Check sheet for the modelled part. Datum: model origin and axes. Units: mm. A direction names the side the tool comes from. Give positions to 0.01 mm unless a question says otherwise; leave off trailing zeros. Order: outer loops, then holes, each group sorted by start corner. A loop starts at its lowest first (then second) coordinate and runs counter-clockwise, first axis right, second up.
Autodesk Inventor part; units mm, degrees
ref_plane "YZ Plane" through (0, 0, 0) normal (1, 0, 0) x (0, 1, 0)
ref_plane "XZ Plane" through (0, 0, 0) normal (0, 1, 0) x (-1, 0, 0)
ref_plane "XY Plane" through (0, 0, 0) normal (0, 0, 1) x (1, 0, 0)
sketch "스케치1" plane through (0, 0, 0) normal (0, 1, 0) x (-1, 0, 0)
  line L0 (-21.65, 75) -> (21.65, 75)
  line L1 (21.65, 75) -> (21.65, -75)
  line L2 (21.65, -75) -> (-21.65, -75)
  line L3 (-21.65, -75) -> (-21.65, 75)
  line L4 (-21.65, 75) -> (21.65, -75) construction
  line L5 (21.65, 75) -> (-21.65, -75) construction
  line L6 (-21.65, 7) -> (21.65, 7)
  point P0 (0, 0)
  dimension "d0" = 43.3
  dimension "d1" = 150
  dimension "d2" = 68
extrude "돌출2" add sketch "스케치1" along normal blind 5 contours L0 L1 L6 L3
extrude "돌출3" add sketch "스케치1" along normal blind 8.5 contours L6 L1 L2 L3
sketch "스케치3" plane through (0, 8.5, 0) normal (0, 1, 0) x (1, 0, 0)
  line L0 (-21.65, -7) -> (21.65, -7)
  line L1 (21.65, 75) -> (-21.65, 75)
  line L2 (6.1, -7) -> (-6.1, -7)
  line L3 (-6.1, -7) -> (-6.1, 75)
  line L4 (-6.1, 75) -> (6.1, 75)
  line L5 (6.1, 75) -> (6.1, -7)
  line L6 (21.65, -7) -> (21.65, 75)
  line L7 (21.65, 75) -> (6.1, 75)
  line L8 (6.1, 75) -> (6.1, -7)
  line L9 (6.1, -7) -> (21.65, -7)
  line L10 (21.65, -7) -> (21.65, 75)
  line L11 (-21.65, 75) -> (-6.1, 75)
  line L12 (-6.1, 75) -> (-6.1, -7)
  line L13 (-6.1, -7) -> (-21.65, -7)
  line L14 (-21.65, -7) -> (-21.65, 75)
  point P0 (0, 0)
  point P1 (-6.1, -7)
  point P2 (6.1, 75)
  dimension "d9" = 12.2
  dimension "d11" = 6.1
extrude "돌출4" add sketch "스케치3" along normal blind 12.2 contours L14 L1 L3 L0 | L5 L1 L6 L0
sketch "스케치4" plane through (0, 5, 0) normal (0, 1, 0) x (1, 0, 0)
  line L0 (16.55, -19.1) -> (16.55, -62.7) construction
  line L1 (14.55, -21.1) -> (14.55, -60.7)
  line L2 (18.55, -60.7) -> (18.55, -21.1)
  arc A0 (18.55, -21.1) -> (14.55, -21.1) centre (16.55, -21.1) ccw
  arc A1 (14.55, -60.7) -> (18.55, -60.7) centre (16.55, -60.7) ccw
  line L3 (21.65, -75) -> (21.65, -7)
  line L4 (-21.65, -75) -> (21.65, -75)
  line L5 (21.65, -7) -> (-21.65, -7)
  line L6 (0, -7) -> (0, -75)
  line L7 (-16.55, -19.1) -> (-16.55, -62.7) construction
  line L8 (-14.55, -21.1) -> (-14.55, -60.7)
  line L9 (-18.55, -60.7) -> (-18.55, -21.1)
  arc A2 (-14.55, -21.1) -> (-18.55, -21.1) centre (-16.55, -21.1) ccw
  arc A3 (-18.55, -60.7) -> (-14.55, -60.7) centre (-16.55, -60.7) ccw
  point P0 (0, 0)
  point P1 (16.55, -40.9)
  point P2 (-16.55, -40.9)
  dimension "d14" = 43.6
  dimension "d15" = 3.1
  dimension "d16" = 4
  dimension "d17" = 12.3
extrude "돌출5" cut sketch "스케치4" against normal through all contours A0 L2 A1 L1 | L8 A3 L9 A2
fillet "모깎기1" radius 4.5 2 edges at (21.65, 2.5, 75) (-21.65, 2.5, 75)
sketch "스케치5" plane through (-21.65, 5, 7) normal (0, 0, 1) x (1, 0, 0)
  line L0 (27.75, 3.5) -> (15.55, 3.5)
  line L1 (21.65, 3.5) -> (21.65, 29.9168)
  line L2 (43.3, 0) -> (43.3, 15.7)
  line L3 (4.5, 0) -> (38.8, 0)
  line L4 (43.3, 15.7) -> (27.75, 15.7)
  line L5 (27.75, 15.7) -> (27.75, 0)
  line L6 (27.75, 0) -> (43.3, 0)
  line L7 (43.3, 0) -> (43.3, 15.7)
  line L8 (43.3, 0) -> (29.75, 15.7)
  line L9 (43.3, 15.7) -> (27.75, 15.7)
  line L10 (43.3, -5) -> (38.8, -5)
  line L11 (0, 0) -> (0, 15.7)
  line L12 (0, 15.7) -> (15.55, 15.7)
  line L13 (0, 0) -> (0, 15.7)
  line L14 (0, 0) -> (13.55, 15.7)
  point P0 (21.65, -5)
  dimension "d21" = 2
  dimension "d22" = 5
extrude "돌출6" cut sketch "스케치5" against normal through all contours L8 L4 L2 | L11 L12 L14
sketch "스케치7" plane through (-21.65, 5, -75) normal (-0.757, 0.6534, 0) x (0, 0, 1)
  line L0 (0, 20.7387) -> (82, 20.7387)
  line L1 (82, 0) -> (0, 0)
  line L2 (82, 20.7387) -> (82, 0)
  circle A0 centre (10, 9.7387) radius 1.75
  line L3 (82, 28.2909) -> (82, 0)
  line L4 (82, 9.7387) -> (0, 9.7387)
  line L5 (0, 24.5057) -> (0, -3.7852)
  line L6 (82, 20.7806) -> (0, 20.7806)
  line L7 (41, 20.7806) -> (41, 0)
  circle A1 centre (72, 9.7387) radius 1.75
  dimension "d26" = 3.5
  dimension "d28" = 10
  dimension "d39" = 11
extrude "돌출7" cut sketch "스케치7" against normal blind 10 contours L4 A0 | A0 L4 | A1 L4 | L4 A1
mirror "미러1" about plane through (0, 0, 0) normal (1, 0, 0) of "돌출7"
sketch "스케치9" plane through (0, 8.5, 0) normal (0, 1, 0) x (1, 0, 0)
  ellipse E0 centre (-15.2871, 3) end of major axis (-15.2871, 1.25) minor radius 1.1434
  ellipse E1 centre (-15.2871, 65) end of major axis (-15.2871, 63.25) minor radius 1.1434
  line L0 (-29.6157, 34) -> (32.1158, 34)
  line L1 (-21.65, -7) -> (-21.65, 75)
  line L2 (21.65, 75) -> (21.65, -7)
  line L3 (-21.65, 13) -> (21.65, 13)
  line L4 (21.65, 13) -> (21.65, 55)
  line L5 (21.65, 55) -> (-21.65, 55)
  line L6 (-21.65, 55) -> (-21.65, 13)
  line L7 (-21.65, 75) -> (-21.65, -70.5)
  line L8 (21.65, -70.5) -> (21.65, 75)
  line L9 (-21.65, 24) -> (21.65, 24)
  line L10 (21.65, 24) -> (21.65, 44)
  line L11 (21.65, 44) -> (-21.65, 44)
  line L12 (-21.65, 44) -> (-21.65, 24)
  point P0 (0, 0)
  point P1 (21.65, 13)
  point P2 (-21.65, 44)
  dimension "d32" = 10
  dimension "d33" = 10
  dimension "d36" = 20
  dimension "d38" = 11
extrude "돌출8" cut sketch "스케치9" along normal through all contours L9 L2 L3 L1 | L1 L5 L2 L11
properties part number "sun2" material "티타늄"
(1) Sectioned sample at A-A (z = 41.5). Enter the section's corners in (x, y).
(2) Sectioned sample at B-B (y = 17). Enter the section's corners in (x, z), plus the area to 3 significant figures.
(3) Sectioned sample at D-D (z = -21). Enter the section's corners in (x, y).
(4) Tool access check on faces 1 (the face through (-11, 13, -24)), 2 (the face through (0, 8.5, -33)), 3 (the face through (6.1, 15, -65)), 4 (the face through (-7.699, 5.855, -65.024)). Record the directions out of +Z, -Z, +X, -X, +Y, -Y that give a thin tool (end or side, any length) a straight path to the whole face; none if there is none.
(5) Release check for a two-part mould opening along Z. For faces 5 (the face through (16.6, 2.5, 19.1)), 6 (the face through (0, 8, 7)), 7 (the face through (-6.1, 15, -34)) record: released by +Z, released by -Z, zero draft, split by the parting line, or undercut.
(6) Go/stop test with flat-tipped pins: P1, Ø3, axis at x = 12, y = 13, coming from the +Z side; P2, Ø21.5, axis at x = -4, z = 55, coming from the +Y side; P3, Ø2, axis at y = 16, z = -55.5, coming from the +X side. Record where each tip stops, or that it passes through.
(7) Thickness scan on L1, parallel to X at y = 1.25, z = 60; L2, parallel to Z at x = -12.5, y = 15.5; L3, parallel to Z at x = 17.5, y = 6.75. Record the ranges inside material, lowest first.
(8) Sectioned sample at C-C (x = 4). Enter the section's corners in (y, z).
Values follow:
1. outline: (-21.65, 0) - (-18.55, 0) - (-18.55, 5) - (-21.65, 5) - close; (-14.55, 0) - (14.55, 0) - (14.55, 5) - (-14.55, 5) - close; (18.55, 0) - (21.65, 0) - (21.65, 5) - (18.55, 5) - close
2. outline: (-11.29, -75) - (-6.1, -75) - (-6.1, -55) - (-11.29, -55) - close; (-11.29, -44) - (-6.1, -44) - (-6.1, -24) - (-11.29, -24) - close; (-11.29, -13) - (-6.1, -13) - (-6.1, 7) - (-11.29, 7) - close; (6.1, -75) - (11.29, -75) - (11.29, -55) - (6.1, -55) - close; (6.1, -44) - (11.29, -44) - (11.29, -24) - (6.1, -24) - close; (6.1, -13) - (11.29, -13) - (11.29, 7) - (6.1, 7) - close
2. area: 623 mm2
3. outline: (-21.65, 0) - (21.65, 0) - (21.65, 5) - (18.63, 8.5) - (-18.63, 8.5) - (-21.65, 5) - close
4. face 1: +X, -X, +Y
4. face 2: +Y
4. face 3: +Z, -Z, +Y
4. face 4: none
5. face 5: undercut
5. face 6: released by +Z
5. face 7: zero draft
6. P1: stops at z = 7
6. P2: stops at y = 5
6. P3: stops at x = 13.02
7. L1: x = -21.65 to -18.55, -14.55 to 14.55, 18.55 to 21.65
7. L2: z = -75 to -55, -44 to -24, -13 to 7
7. L3: z = -75 to 7
8. outline: (0, -75) - (8.5, -75) - (8.5, 7) - (5, 7) - (5, 75) - (0, 75) - close
